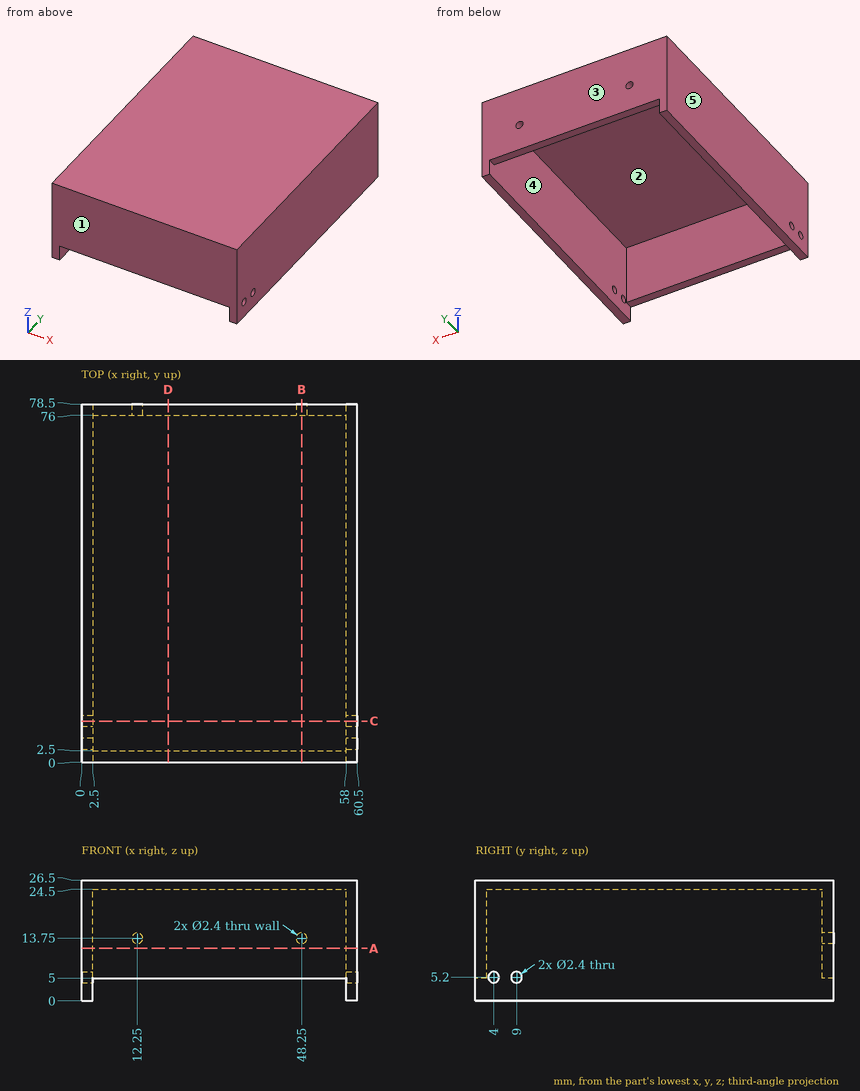
Verification items for this drawing (mm, ordinates from the low corner). A direction names the side the tool comes from. Give positions to 0.01 mm unless a question says otherwise; leave off trailing zeros. Write each loop counter-clockwise with the first axis right and the second up, starting at its lowest first coordinate (ties: lowest second). Pieces come first, ordered by that corner, then holes. Notation, with made-up numbers: (53, -35) - (86, -35) arc R20 cw to (86, -14) - close; hole circle Ø7 at (39.25, 49.25). An arc over 180 degrees is marked (long way). Answer as a JSON object with one key per item and string values. Group by question number.
1) Thickness scan on probe 1 along Y at (x, z) = (10, 14.25); probe 2 along X at (y, z) = (38, 6); probe 3 along Z at (x, y) = (48.25, 76.95). Record the ranges inside material, lowest first. Write a range as from..to.
2) Access from +Z, -Z, +X, -X, +Y, -Y to the whole of each face (thin tool, end or side, straight path). Record for the marked faces 4 and 5.
3) Sectioned sample at B-B (x = 48.25). Record the cut outline in (y, z).
4) Sectioned sample at C-C (y = 9). Record the cut outline in (x, z).
5) Depth check by flat-ended pin: P1, Ø16.5, axis at x = 39, y = 40.5, coming from the -Z side; P2, Ø2, axis at x = 38, y = 1, coming from the -Z side; P3, Ø1.9, axis at x = 12.25, z = 13.75, coming from the +Y side. Enter the tip coordinate at first touch or a pass-through.
6) Sectioned sample at A-A (z = 11.5). Record the cut outline in (x, y), then the cut area to 3 significant figures.
7) Release check for a two-part mould opening along Y. For the marked faces 1, 2 and 3 record: pulls with the +Y half, pulls with the -Y half, needs draft (parallel to the pull), parting line crosses it, or undercut.
8) Sectioned sample at D-D (x = 19). Record the cut outline in (y, z).
Geometry results:
{
 "1": {"probe 1": "y = 0..2.5, 76..78.5", "probe 2": "x = 0..2.5, 58..60.5", "probe 3": "z = 5..12.55, 14.95..26.5"},
 "2": {"face 4": "-Z", "face 5": "+Z, -Z, -X, +Y, -Y"},
 "3": {"outline": "(0, 5) - (2.5, 5) - (2.5, 24.5) - (76, 24.5) - (76, 14.95) - (78.5, 14.95) - (78.5, 26.5) - (0, 26.5) - close; (76, 5) - (78.5, 5) - (78.5, 12.55) - (76, 12.55) - close"},
 "4": {"outline": "(0, 0) - (2.5, 0) - (2.5, 4) - (0, 4) - close; (0, 6.4) - (2.5, 6.4) - (2.5, 24.5) - (58, 24.5) - (58, 6.4) - (60.5, 6.4) - (60.5, 26.5) - (0, 26.5) - close; (58, 0) - (60.5, 0) - (60.5, 4) - (58, 4) - close"},
 "5": {"P1": "stops at z = 24.5", "P2": "stops at z = 5", "P3": "stops at y = 2.5"},
 "6": {"outline": "(0, 0) - (60.5, 0) - (60.5, 78.5) - (0, 78.5) - close; hole (2.5, 2.5) - (58, 2.5) - (58, 76) - (2.5, 76) - close", "area": "670 mm^2"},
 "7": {"face 1": "pulls with the -Y half", "face 2": "undercut", "face 3": "pulls with the +Y half"},
 "8": {"outline": "(0, 5) - (2.5, 5) - (2.5, 24.5) - (76, 24.5) - (76, 5) - (78.5, 5) - (78.5, 26.5) - (0, 26.5) - close"}
}
